```python
from build123d import *

# Parameters (mm, degrees)
BOSS_EXTRUDE1_DEPTH = 3.175
CUT_EXTRUDE1_DEPTH  = 4.175
CUT_EXTRUDE2_DEPTH  = 7.62


with BuildPart() as part:
    # Sketch1 → Boss-Extrude1 (new body)
    with BuildSketch(Plane.XY):
        Polygon((-950.530495659, 69.619322302), (-951.061849964, 63.291592645), (-11.536706102, -24.902638492), (-8.372841274, -25.168315645), (0, -25.545856054), (152.4, -25.545856054), (152.4, -7.765856054), (139.7, -7.765856054), (139.7, -12.845856054), (136.525, -12.845856054), (136.525, -7.765856054), (95.25, -7.765856054), (95.25, -12.845856054), (92.075, -12.845856054), (92.075, -7.765856054), (79.375, -7.765856054), (79.375, -12.845856054), (76.2, -12.845856054), (76.2, -7.765856054), (69.85, -7.765856054), (25.4, -0.145856054), (19.05, -0.145856054), (19.05, -5.225856054), (15.875, -5.225856054), (15.875, -0.145856054), (3.175, -0.145856054), (3.175, -6.495856054), (0, -6.495856054), (0, -0.145856054), (-2.81225704, -0.145856054), (-6.247424053, 0.14260298), (-6.778778359, -6.185126677), (-9.942643187, -5.919449524), (-9.411288881, 0.408280132), (-946.54805097, 79.101852726), (-947.366630831, 69.353645149), align=None)
    extrude(amount=BOSS_EXTRUDE1_DEPTH)

    # Sketch2 → Cut-Extrude1 (cut, through all)
    with BuildSketch(Plane.XY.offset(3.175)):
        Polygon((-869.047169109, 67.116306724), (-868.590421605, 72.555567687), (-871.754286433, 72.821244839), (-872.210759203, 67.385255598), align=None)
        Polygon((-790.083960364, 60.403342827), (-789.620355495, 65.924265958), (-792.784220323, 66.189943111), (-793.247550458, 60.672291701), align=None)
        Polygon((-711.120751618, 53.69037893), (-710.650289385, 59.29296423), (-713.814154213, 59.558641383), (-714.284341712, 53.959327804), align=None)
        Polygon((-632.157542872, 46.977415032), (-631.680223276, 52.661662502), (-634.844088104, 52.927339654), (-635.321132966, 47.246363906), align=None)
        Polygon((-553.194334126, 40.264451135), (-552.710157166, 46.030360773), (-555.874021994, 46.296037926), (-556.35792422, 40.533400009), align=None)
        Polygon((-474.23112538, 33.551487238), (-473.740091056, 39.399059045), (-476.903955884, 39.664736197), (-477.394715474, 33.820436112), align=None)
        Polygon((-395.267916634, 26.83852334), (-394.770024946, 32.767757316), (-397.933889774, 33.033434469), (-398.431506728, 27.107472214), align=None)
        Polygon((-316.304707888, 20.125559443), (-315.799958836, 26.136455588), (-318.963823664, 26.402132741), (-319.468297982, 20.394508317), align=None)
        Polygon((-237.341499142, 13.412595546), (-236.829892727, 19.50515386), (-239.993757555, 19.770831012), (-240.505089236, 13.68154442), align=None)
        Polygon((-158.378290396, 6.699631648), (-157.859826617, 12.873852131), (-161.023691445, 13.139529284), (-161.54188049, 6.968580522), align=None)
        Polygon((-79.415081651, -0.013332249), (-78.889760507, 6.242550403), (-82.053625335, 6.508227555), (-82.578671745, 0.255616625), align=None)
    extrude(amount=-CUT_EXTRUDE1_DEPTH, mode=Mode.SUBTRACT)

    # Sketch3 → Cut-Extrude2 (cut)
    with BuildSketch(Plane.XY.offset(3.175)):
        Polygon((-435.836990415, 36.216246757), (-435.836990415, 26.451619727), (-427.115588921, 26.451619727), (-427.115588921, 14.108196169), (150.838987184, -84.054223576), (191.196568658, 26.451619727), align=None)
    extrude(amount=-CUT_EXTRUDE2_DEPTH, mode=Mode.SUBTRACT)


solid = part.part
```
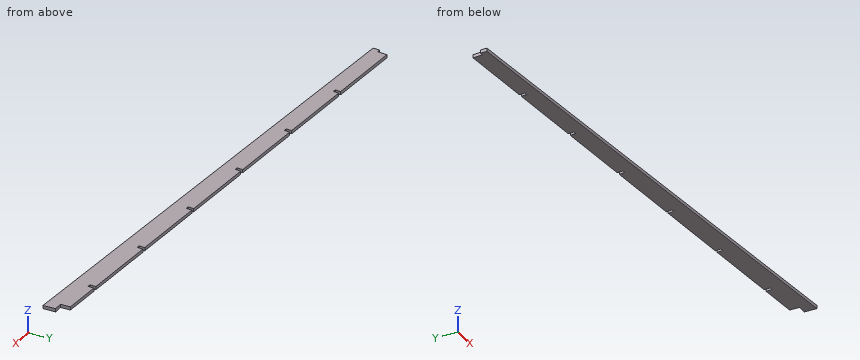
For this review, take the finished solid that the model builds, in its own axes (mm). Give positions to 0.01 mm unless a question says otherwise; leave off trailing zeros. Write each loop counter-clockwise with the first axis right and the second up, starting at its lowest first coordinate (ties: lowest second). Pieces come first, ordered by that corner, then holes.
Item 1: Take a section at B-B (x = -918.5). Give the boundary of the cut face in (y, z) (3 decimals), and give its area (3 significant figures).
Item 2: Insertion check: P1, Ø1.6, axis at y = 32, z = 1, coming from the +X side; P2, Ø1.5, axis at x = -696, z = 2, coming from the -Y side. Each pin has a flat end and moves straight along its axis. Give the tip position at first contact, or say it passes through.
Item 3: Wall thickness on probe 1 along Y at (x, z) = (-626, 0.8); probe 2 along Y at (x, z) = (-699.5, 1.7): over which ranges is each line inside the solid? List them lowest first.
Item 4: Take a section at C-C (x = -849). Give the boundary of the cut face in (y, z) (3 decimals).
Established:
1. outline: (60.235, 0) - (76.747, 0) - (76.747, 3.175) - (60.235, 3.175) - close
1. area: 52.4 mm2
2. P1: stops at x = -435.84
2. P2: stops at y = 39.28
3. probe 1: y = 32.78 to 52.18
3. probe 2: y = 39.68 to 58.36
4. outline: (53.711, 0) - (70.911, 0) - (70.911, 3.175) - (53.711, 3.175) - close
